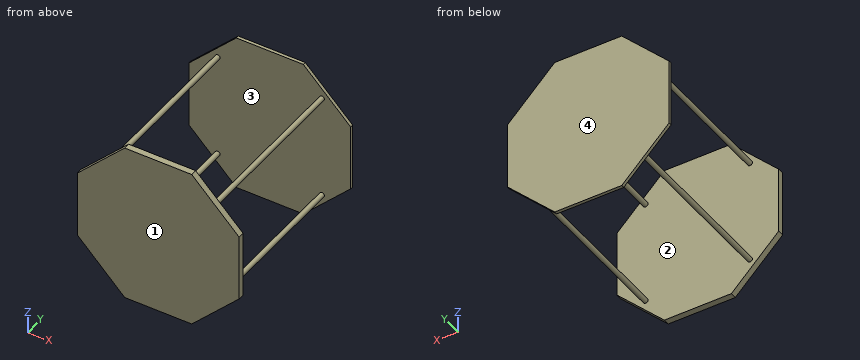
```python
from build123d import *

# Parameters (mm, degrees)
BOSS_EXTRUDE1_DEPTH = 6.35
SKETCH2_R           = 2.54
BOSS_EXTRUDE2_DEPTH = 173.863
BOSS_EXTRUDE3_DEPTH = 3.175


with BuildPart() as part:
    # Sketch1 → Boss-Extrude1 (new body)
    with BuildSketch(Plane(origin=(0, 0, 0), x_dir=(1, 0, 0), z_dir=(0, 1, 0))):
        Polygon((34.248980878, -82.684354133), (82.684354133, -34.248980878), (82.684354133, 34.248980878), (34.248980878, 82.684354133), (-34.248980878, 82.684354133), (-82.684354133, 34.248980878), (-82.684354133, -34.248980878), (-34.248980878, -82.684354133), align=None)
    extrude(amount=BOSS_EXTRUDE1_DEPTH)

    # Sketch2 → Boss-Extrude2 (add)
    with BuildSketch(Plane(origin=(0, 6.35, 0), x_dir=(1, 0, 0), z_dir=(0, 1, 0))):
        with Locations(Location((53.34, 53.34, 0), (0, 0, 270))):
            Circle(SKETCH2_R)
        with Locations(Location((-53.34, 53.34, 0), (0, 0, 90))):
            Circle(SKETCH2_R)
        with Locations(Location((53.34, -53.34, 0), (0, 0, 90))):
            Circle(SKETCH2_R)
        with Locations(Location((-53.34, -53.34, 0), (0, 0, 270))):
            Circle(SKETCH2_R)
    extrude(amount=BOSS_EXTRUDE2_DEPTH)

    # Sketch3 → Boss-Extrude3 (add)
    with BuildSketch(Plane(origin=(0, 180.213, 0), x_dir=(1, 0, 0), z_dir=(0, 1, 0))):
        Polygon((82.684354133, -34.248980878), (82.684354133, 34.248980878), (34.248980878, 82.684354133), (-34.248980878, 82.684354133), (-82.684354133, 34.248980878), (-82.684354133, -34.248980878), (-34.248980878, -82.684354133), (34.248980878, -82.684354133), align=None)
    extrude(amount=BOSS_EXTRUDE3_DEPTH)


solid = part.part
```
CAD build for the part. Positions are in the model's coordinates, mm. Face numbers are marked on the shaded views. Coordinates: 2 decimals unless noted, no trailing zeros. Loops run counter-clockwise (first coordinate to the right, second up) from the corner with the lowest first, then second, coordinate; pieces in that order, holes last. Notation, with made-up numbers: (-19, 35) - (35, 35) arc R26 cw to (35, 58) - close; hole circle Ø1 at (70.25, 78). An arc over 180 degrees is marked (long way). Use CSV: the item, a comma, the result in double quotes. Start each with the question number.
Q1. Probe probe 1 along Y at (x, z) = (38.5, -45); probe 2 along Z at (x, y) = (53, 113.5); probe 3 along Z at (x, y) = (55, 63). List the from-to ranges inside material, lowest first. Write a range as from..to.
Q2. Cut at D-D, the plane y = 66. List the corners of the cut face in (x, z).
Q3. Two-plate mould, pull along Y, no slides. Class the marked faces 1, 2, 3 and 4: +Y half, -Y half, draft (parallel to the pull), parting line (faces both ways), or undercut.
Q4. Cut at B-B, the plane x = -12. List the corners of the cut face in (y, z).
Q5. Drop a flat-ended pin along its axis: P1, Ø10, axis at x = 57, y = 85.5, coming from the +Z side. Give the stop position or say it passes through.
Q6. Cut at C-C, the plane x = 53.34. List the corners of the cut face in (y, z), then the cut area to 3 significant figures.
Q7. Cut at A-A, the plane z = -20. List the corners of the cut face in (x, y), then the cut area to 3 significant figures.
Here are the results:
1,probe 1,"0..6.35, 180.21..183.39"
1,probe 2,"-55.86..-50.82, 50.82..55.86"
1,probe 3,"-55.26..-51.42, 51.42..55.26"
2,outline,"circle Ø5.08 at (-53.34, -53.34); circle Ø5.08 at (-53.34, 53.34); circle Ø5.08 at (53.34, -53.34); circle Ø5.08 at (53.34, 53.34)"
3,face 1,"-Y half"
3,face 2,"undercut"
3,face 3,"undercut"
3,face 4,"+Y half"
4,outline,"(0, -82.68) - (6.35, -82.68) - (6.35, 82.68) - (0, 82.68) - close; (180.21, -82.68) - (183.39, -82.68) - (183.39, 82.68) - (180.21, 82.68) - close"
5,P1,"z = 55.88"
6,outline,"(0, -63.59) - (6.35, -63.59) - (6.35, -55.88) - (180.21, -55.88) - (180.21, -63.59) - (183.39, -63.59) - (183.39, 63.59) - (180.21, 63.59) - (180.21, 55.88) - (6.35, 55.88) - (6.35, 63.59) - (0, 63.59) - close; hole (6.35, -50.8) - (180.21, -50.8) - (180.21, 50.8) - (6.35, 50.8) - close"
6,area,"2,980 mm2"
7,outline,"(-82.68, 0) - (82.68, 0) - (82.68, 6.35) - (-82.68, 6.35) - close; (-82.68, 180.21) - (82.68, 180.21) - (82.68, 183.39) - (-82.68, 183.39) - close"
7,area,"1,580 mm2"
